Autodesk Inventor part; units mm, degrees
ref_plane "YZ Plane" through (0, 0, 0) normal (1, 0, 0) x (0, 1, 0)
ref_plane "XZ Plane" through (0, 0, 0) normal (0, 1, 0) x (-1, 0, 0)
ref_plane "XY Plane" through (0, 0, 0) normal (0, 0, 1) x (1, 0, 0)
sketch "Sketch1" plane through (0, 0, 0) normal (0, 1, 0) x (-1, 0, 0)
  line L0 (101.6, -101.6) -> (-101.6, -101.6)
  line L1 (-101.6, -101.6) -> (-101.6, 101.6)
  line L2 (-101.6, 101.6) -> (101.6, 101.6)
  line L3 (101.6, 101.6) -> (101.6, -101.6)
  line L4 (96.6, -96.6) -> (-96.6, -96.6)
  line L5 (-96.6, -96.6) -> (-96.6, 96.6)
  line L6 (-96.6, 96.6) -> (96.6, 96.6)
  line L7 (96.6, 96.6) -> (96.6, -96.6)
  line L8 (101.6, 101.6) -> (-40.4, 101.6)
  circle A0 centre (0, 0) radius 88.9
  line L9 (-40.4, 101.6) -> (-101.6, 40.4)
  line L10 (-45.4, 101.6) -> (-101.6, 45.4)
  line L11 (96.6, 96.6) -> (96.6, 101.6)
  line L12 (-45.4, 101.6) -> (-35.4, 101.6)
  line L13 (-35.4, 101.6) -> (-35.4, 96.6)
  line L14 (-35.4, 96.6) -> (-45.4, 96.6)
  line L15 (-45.4, 96.6) -> (-45.4, 101.6)
  line L16 (-101.6, 39.4) -> (-39.4, 101.6)
  line L17 (96.4, -96.4) -> (-96.4, -96.4)
  line L18 (-96.4, -96.4) -> (-96.4, 96.4)
  line L19 (-96.4, 96.4) -> (96.4, 96.4)
  line L20 (96.4, 96.4) -> (96.4, -96.4)
  circle A1 centre (0, 0) radius 90.9
  point P0 (96.6, 51.2168)
  point P1 (101.6, 40.4)
  point P2 (101.6, -40.4)
  point P3 (96.6, -51.2168)
  point P4 (-96.6, 45.4)
  point P5 (-45.4, 96.6)
  point P6 (-44.6, 96.4)
  point P7 (-96.4, 44.6)
  dimension "d0" = 203.2
  dimension "d1" = 203.2
  dimension "d2" = 101.6
  dimension "d3" = 101.6
  dimension "d4" = 5
  dimension "d5" = 5
  dimension "d6" = 5
  dimension "d7" = 5
  dimension "d8" = 142
  dimension "d9" = 61.2
  dimension "d10" = 177.8
  dimension "d11" = 5
  dimension "d12" = 5
  dimension "d13" = 10
  dimension "d14" = 1
  dimension "d15" = 0.2
  dimension "d16" = 0.2
  dimension "d17" = 0.2
  dimension "d18" = 0.2
  dimension "d64" = 181.8
extrude "Extrusion1" add sketch "Sketch1" along normal blind 4 contours L16 L19 L20 L17 L18
sketch "Sketch6" plane through (0, 4, 0) normal (0, 1, 0) x (1, 0, 0)
  line L0 (96.4, 96.4) -> (-96.4, 96.4)
  line L1 (96.4, 96.4) -> (88.4, 96.4)
  line L2 (88.4, 96.4) -> (88.4, -45.6)
  line L3 (88.4, -45.6) -> (96.4, -45.6)
  line L4 (96.4, -45.6) -> (96.4, 96.4)
  line L5 (96.4, -44.6) -> (96.4, 96.4)
  line L6 (88.4, -12) -> (96.4, -12)
  line L7 (96.4, -12) -> (96.4, 12)
  line L8 (96.4, 12) -> (88.4, 12)
  line L9 (88.4, 12) -> (88.4, -12)
  line L10 (0, 0) -> (96.4, 0)
  point P0 (96.4, -12)
  dimension "d58" = 8
  dimension "d59" = 142
  dimension "d62" = 12
  dimension "d63" = 12
extrude "Extrusion6" cut sketch "Sketch6" against normal blind 25.4 contours L4 L10 L2 L8 | L4 L6 L2 L10
sketch "Sketch8" plane through (0, 4, 0) normal (0, 1, 0) x (1, 0, 0)
  line L0 (-96.6, 96.6) -> (-96.6, -96.6)
  line L1 (96.6, 96.6) -> (-96.6, 96.6)
  line L2 (-96.6, 96.6) -> (96.6, 96.6)
  line L3 (96.6, -45.4) -> (45.4, -96.6)
  line L4 (96.6, 96.6) -> (96.6, -45.4)
  line L5 (96.6, -45.4) -> (45.4, -96.6)
  line L6 (45.4, -96.6) -> (-96.6, -96.6)
  line L7 (-96.6, -96.6) -> (-96.6, 96.6)
  line L8 (-96.6, 96.6) -> (-89.5289, 89.5289)
  circle A0 centre (-89.5289, 89.5289) radius 5
  circle A1 centre (-89.5289, 89.5289) radius 1.5
  line L9 (-89.5289, 84.5289) -> (-96.6, 84.5289)
  line L10 (-89.5289, 89.5289) -> (-89.5289, 84.5289)
  line L11 (-89.5289, 89.5289) -> (-84.5289, 89.5289)
  line L12 (-84.5289, 96.6) -> (-84.5289, 89.5289)
  line L13 (-96.6, -96.6) -> (-89.5289, -89.5289)
  line L14 (-96.6, -96.6) -> (-86.6, -96.6) construction
  circle A2 centre (-89.5289, -89.5289) radius 5
  circle A3 centre (-89.5289, -89.5289) radius 1.75
  line L15 (-89.5289, -89.5289) -> (-84.5289, -89.5289)
  line L16 (-84.5289, -96.6) -> (-84.5289, -89.5289)
  line L17 (-89.5289, -89.5289) -> (-89.5289, -84.5289)
  line L18 (-96.6, -84.5289) -> (-89.5289, -84.5289)
  line L19 (96.6, 96.6) -> (89.5289, 89.5289)
  circle A4 centre (89.5289, 89.5289) radius 5
  circle A5 centre (89.5289, 89.5289) radius 1.75
  line L20 (89.5289, 89.5289) -> (84.5289, 89.5289)
  line L21 (84.5289, 96.6) -> (84.5289, 89.5289)
  line L22 (89.5289, 89.5289) -> (89.5289, 84.5289)
  line L23 (96.6, 84.5289) -> (89.5289, 84.5289)
  line L24 (96.6, -43.114) -> (96.6, 96.6)
  line L25 (-96.6, -96.6) -> (43.1178, -96.6)
  line L26 (28.9914, 5.6569) -> (-5.6569, -28.9914)
  line L27 (25.4, -25.4) -> (101.6, -25.4)
  line L28 (101.6, -88.9) -> (101.6, 101.6)
  line L29 (25.4, -25.4) -> (25.4, -101.6)
  line L30 (43.1178, -101.6) -> (-101.6, -101.6)
  line L31 (96.6, -25.4) -> (86.6, -25.4)
  circle A6 centre (86.6, -25.4) radius 5
  circle A7 centre (86.6, -25.4) radius 1.75
  line L32 (25.4, -96.6) -> (25.4, -86.6)
  circle A8 centre (25.4, -86.6) radius 5
  circle A9 centre (25.4, -86.6) radius 1.75
  line L33 (44.6, -96.4) -> (96.4, -44.6)
  circle A10 centre (68.7322, -68.7322) radius 1
  point P0 (0, 0)
  point P1 (0, 0)
  point P2 (0, 0)
  dimension "d90" = 10
  dimension "d91" = 3
  dimension "d92" = 10
  dimension "d93" = 45
  dimension "d94" = 10
  dimension "d95" = 3.5
  dimension "d96" = 10
  dimension "d97" = 10
  dimension "d98" = 3.5
  dimension "d99" = 76.2
  dimension "d100" = 76.2
  dimension "d101" = 10
  dimension "d102" = 10
  dimension "d103" = 3.5
  dimension "d104" = 10
  dimension "d105" = 10
  dimension "d106" = 3.5
  dimension "d115" = 2
  dimension "d116" = 2.5
hole "Hole1" at (-89.5289, 4, -89.5289) at (89.5289, 4, -89.5289) at (-89.5289, 4, 89.5289) at (68.7322, 4, 68.7322) direction (0, -1, 0) diameter 3.1211 depth 2.75 tip angle 118 countersink diameter 3.2004 countersink angle 82
fillet "Fillet1" radius 3.175 2 edges at (-6.0132, 0, -90.7009) (-6.0132, 0, 90.7009)
sketch "Sketch9" plane through (0, 4, 0) normal (0, 1, 0) x (1, 0, 0)
  arc A0 (-101.6, -98.425) -> (-98.425, -101.6) centre (-98.425, -98.425) ccw
  line L0 (44.0849, 101.6) -> (-98.425, 101.6)
  line L1 (-101.6, 98.425) -> (-101.6, -98.425)
  line L2 (-101.6, -46.1) -> (-101.6, -76.6)
  line L3 (-96.6, -96.6) -> (-96.6, 96.6)
  line L4 (-96.6, -46.1) -> (-96.6, -76.6)
  line L5 (-101.6, -76.6) -> (-96.6, -76.6)
  line L6 (-101.6, -46.1) -> (-96.6, -46.1)
  line L7 (-98.425, -101.6) -> (101.6, -101.6)
  line L8 (0, 0) -> (-101.6, 0)
  line L9 (-101.6, 46.1) -> (-101.6, 76.6)
  line L10 (-96.6, 46.1) -> (-96.6, 76.6)
  line L11 (-101.6, 76.6) -> (-96.6, 76.6)
  line L12 (-101.6, 46.1) -> (-96.6, 46.1)
  line L13 (-96.6, -76.6) -> (-90.1, -76.6)
  line L14 (-90.1, -76.6) -> (-90.1, -46.1)
  line L15 (-90.1, -46.1) -> (-96.6, -46.1)
  line L16 (-96.6, -46.1) -> (-96.6, -76.6)
  arc A1 (-98.425, 101.6) -> (-101.6, 98.425) centre (-98.425, 98.425) ccw
  line L17 (-101.6, 46.1) -> (-96.6, 46.1)
  line L18 (-90.1, 46.1) -> (-96.6, 46.1)
  line L19 (-101.6, 46.1) -> (-101.6, 76.6)
  line L20 (-96.6, 46.1) -> (-96.6, 76.6)
  line L21 (-96.6, 46.1) -> (-96.6, 76.6)
  line L22 (-90.1, 76.6) -> (-90.1, 46.1)
  line L23 (-101.6, 76.6) -> (-96.6, 76.6)
  line L24 (-96.6, 76.6) -> (-90.1, 76.6)
  point P0 (-98.425, 98.425)
  point P1 (46.1, 101.6)
  point P2 (46.1, 96.6)
  point P3 (76.6, 96.6)
  point P4 (76.6, 101.6)
  point P5 (-46.1, 96.6)
  dimension "d117" = 30.5
  dimension "d118" = 25
  dimension "d119" = 6.5
extrude "Extrusion7" cut sketch "Sketch9" against normal blind 25.4 contours L24 L22 L18 L3 | L15 L14 L13 L3
sketch "Sketch10" plane through (0, 4, 0) normal (0, 1, 0) x (1, 0, 0)
  line L0 (-96.3514, 0) -> (-90.9, 0)
  arc A0 (90.1044, 12) -> (90.1044, -12) centre (0, 0) ccw
ref_plane "Work Plane1" through (-96.3514, 4, 0) normal (0, 0, 1) x (1, 0, 0)
sketch "Sketch11" plane through (-96.3514, 4, 0) normal (0, 0, 1) x (1, 0, 0)
  line L0 (-51.1439, 37.1405) -> (237.6314, 37.1405)
  line L1 (237.6314, 37.1405) -> (237.6314, -59.6996)
  line L2 (237.6314, -59.6996) -> (-51.1439, -59.6996)
  line L3 (-51.1439, -59.6996) -> (-51.1439, 37.1405)
  point P0 (96.3514, -4)
extrude "Extrusion8" cut sketch "Sketch11" against normal through all
equation "\"d1\" = d0"
equation "\"d15\" = d17"
equation "\"d16\" = d17"
equation "\"d18\" = d17"
properties part number "Drop_Plate"
Input: part model. Units: mm. Frame: model coordinates. A direction names the side the tool comes from. Round coordinates to 2 decimals unless told otherwise and drop trailing zeros. Loops run counter-clockwise (first coordinate to the right, second up) from the corner with the lowest first, then second, coordinate; pieces in that order, holes last. Notation, with made-up numbers: (8.5, 10.5) -> (53.5, 10.5) arc R13 ccw to (53.5, 29.5) -> close; hole circle Ø6 at (12, -21.5). An arc over 180 degrees is marked (long way). One line per item, written item: value.
(1) Section A-A (x = 0). Return the cut outline in (y, z) (3 decimals).
Geometry check:
outline: (0, 94.075) arc R3.175 ccw to (3.175, 90.9) -> (4, 90.9) -> (4, 96.4) -> (0, 96.4) -> close
(2) Material intervals for line 1 (X direction, y = 2.35, z = 36.5); line 2 (X direction, y = 1.3, z = 19); line 3 (Z direction, x = 17, y = 1.1), sorted ascending. Write a range as [from, to].
Geometry check:
line 1: [-96.4, -83.37], [83.37, 96.4]
line 2: [-96.4, -89.52], [89.52, 96.4]
line 3: [90.08, 96.4]
(3) Mould query, pull axis Z, two halves, no side actions, for faces 1 (the face through (71, 2, 70)), 2 (the face through (-28, 4, 88)), 3 (the face through (-93, 2, 76.6)). Classes: pulls with the +Z half, pulls with the -Z half, needs draft (parallel to the pull), parting line crosses it, or undercut.
Geometry check:
face 1: pulls with the +Z half
face 2: needs draft
face 3: undercut
(4) Pin query (flat end, axial travel): pin 1 (1 mm diameter, centred on x = 1, y = 2, fed in from -Z); pin 2 (1.2 mm diameter, centred on y = 2, z = 67, fed in from -X). Return the tip coordinate at first contact, or that it passes through.
Geometry check:
pin 1: z = 90.97
pin 2: x = -90.1
(5) Set-up query: faces 4 (the face through (-93, 2, 46.1)), 5 (the face through (-35, 0, 88)), 6 (the face through (93, 2, 12)). Return all of +Z, -Z, +X, -X, +Y, -Y with unobstructed straight access to the full face (end or side cutting, diameter ignored); none if empty.
Geometry check:
face 4: -X, +Y, -Y
face 5: +Z, -Z, +X, -X, -Y
face 6: -Z, +X, +Y, -Y
